Here's how the part is built. I have some questions about the finished solid (model axes, mm). Coordinates: 2 decimals unless noted, no trailing zeros. Order: outer loops, then holes, each group sorted by start corner. A loop starts at its lowest first (then second) coordinate and runs counter-clockwise, first axis right, second up.
```python
from build123d import *

# Parameters (mm, degrees)
SKETCH1_R           = 35
SKETCH1_R_2         = 28.575
BOSS_EXTRUDE1_DEPTH = 3.18
SKETCH2_R           = 1.47
CUT_EXTRUDE1_DEPTH  = 3.18
CIRPATTERN1_COUNT   = 4


with BuildPart() as part:
    # Sketch1 → Boss-Extrude1 (new body)
    with BuildSketch(Plane.XY):
        with Locations(Location((0, 0, 0), (0, 0, 180))):
            Circle(SKETCH1_R)
        with Locations(Location((0, 0, 0), (0, 0, 180))):
            Circle(SKETCH1_R_2, mode=Mode.SUBTRACT)
    extrude(amount=BOSS_EXTRUDE1_DEPTH)

    # Sketch2 → Cut-Extrude1 (cut)
    with BuildSketch(Plane.XY.offset(3.18)):
        with Locations((0, 33)):
            Circle(SKETCH2_R)
    cut_extrude1 = extrude(amount=-CUT_EXTRUDE1_DEPTH, mode=Mode.SUBTRACT)

    # CirPattern1: Cut-Extrude1 ×4 about axis
    cirpattern1_axis = Axis((0, 0, 0), (0, 0, 1))
    for i in range(1, CIRPATTERN1_COUNT):
        add(cut_extrude1.rotate(cirpattern1_axis, i * 360 / CIRPATTERN1_COUNT), mode=Mode.SUBTRACT)


solid = part.part
```
Q1. I need wall thicknesses on L1, parallel to Y at x = 0, z = 2.3 (3 decimals); L2, parallel to X at y = -20, z = 2.7; L3, parallel to Y at x = 22.5, z = 2.4. Which ranges of each line are inside material? Lowest first, please.
Q2. If we section it at B-B on x = -22.5: Write out the boundary of the cut face in (y, z), then the cut area to 3 significant figures.
Q3. We'd pull the mould along X, two halves only. Please class faces 1 (the cylindrical face through (7.587, 34.168, 1.568)), 2 (the cylindrical face through (31.565, 0.319, 1.612)), 3 (the flat face through (5.3, 28.4, 3.18)): pulls with the +X half, pulls with the -X half, needs draft (parallel to the pull), parting line crosses it, or undercut.
Q4. Will these pins go through, and if not, where does the flat tip stop? pin 1 (1 mm diameter, centred on x = 27.5, z = 1.5, fed in from +Y); pin 2 (4 mm diameter, centred on x = 0, y = -33, fed in from -Z); pin 3 (1.8 mm diameter, centred on x = 33, y = 0, fed in from +Z).
Q5. If we section it at D-D on y = 16.5: Write out the boundary of the cut face in (x, z).
Q6. If we section it at C-C on z = 1.85: Write out the boundary of the cut face in (x, y) (3 decimals).
Q7. If we section it at A-A on y = 0: Write out the boundary of the cut face in (x, z) (3 decimals).
Reply:
1. L1: y = -35 to -34.47, -31.53 to -28.575, 28.575 to 31.53, 34.47 to 35
1. L2: x = -28.72 to -20.41, 20.41 to 28.72
1. L3: y = -26.81 to -17.61, 17.61 to 26.81
2. outline: (-26.81, 0) - (-17.61, 0) - (-17.61, 3.18) - (-26.81, 3.18) - close; (17.61, 0) - (26.81, 0) - (26.81, 3.18) - (17.61, 3.18) - close
2. area: 58.5 mm2
3. face 1: parting line crosses it
3. face 2: undercut
3. face 3: needs draft
4. pin 1: stops at y = 22.27
4. pin 2: stops at z = 0
4. pin 3: passes through
5. outline: (-30.87, 0) - (-23.33, 0) - (-23.33, 3.18) - (-30.87, 3.18) - close; (23.33, 0) - (30.87, 0) - (30.87, 3.18) - (23.33, 3.18) - close
6. outline: circle Ø70 at (0, 0); hole circle Ø2.94 at (-33, 0); hole circle Ø57.15 at (0, 0); hole circle Ø2.94 at (0, -33); hole circle Ø2.94 at (0, 33); hole circle Ø2.94 at (33, 0)
7. outline: (-35, 0) - (-34.47, 0) - (-34.47, 3.18) - (-35, 3.18) - close; (-31.53, 0) - (-28.575, 0) - (-28.575, 3.18) - (-31.53, 3.18) - close; (28.575, 0) - (31.53, 0) - (31.53, 3.18) - (28.575, 3.18) - close; (34.47, 0) - (35, 0) - (35, 3.18) - (34.47, 3.18) - close
